Autodesk Inventor part; units mm, degrees
ref_plane "YZ Plane" through (0, 0, 0) normal (1, 0, 0) x (0, 1, 0)
ref_plane "XZ Plane" through (0, 0, 0) normal (0, 1, 0) x (-1, 0, 0)
ref_plane "XY Plane" through (0, 0, 0) normal (0, 0, 1) x (1, 0, 0)
sketch "Sketch1" plane through (0, 0, 0) normal (0, 1, 0) x (-1, 0, 0)
  line L0 (7.5, 75) -> (-7.5, 75)
  line L1 (-7.5, 75) -> (-7.5, -75)
  line L2 (-7.5, -75) -> (7.5, -75)
  line L3 (7.5, -75) -> (7.5, 75)
  line L4 (-7.5, 75) -> (7.5, -75) construction
  line L5 (-7.5, -75) -> (7.5, 75) construction
  line L6 (7.5, -66.5) -> (9.3, -66.5)
  line L7 (13.3, -70.5) -> (13.3, -71)
  line L8 (9.3, -75) -> (7.5, -75)
  line L9 (7.5, -75) -> (7.5, -66.5)
  arc A0 (13.3, -70.5) -> (9.3, -66.5) centre (9.3, -70.5) ccw
  arc A1 (9.3, -75) -> (13.3, -71) centre (9.3, -71) ccw
  line L10 (0, 75) -> (0, -75) construction
  line L11 (-7.5, -66.5) -> (-9.3, -66.5)
  line L12 (-13.3, -70.5) -> (-13.3, -71)
  line L13 (-9.3, -75) -> (-7.5, -75)
  arc A2 (-9.3, -66.5) -> (-13.3, -70.5) centre (-9.3, -70.5) ccw
  arc A3 (-13.3, -71) -> (-9.3, -75) centre (-9.3, -71) ccw
  line L14 (-7.5, 0) -> (7.5, 0) construction
  line L15 (7.5, 66.5) -> (9.3, 66.5)
  line L16 (13.3, 70.5) -> (13.3, 71)
  line L17 (9.3, 75) -> (7.5, 75)
  arc A4 (9.3, 66.5) -> (13.3, 70.5) centre (9.3, 70.5) ccw
  arc A5 (13.3, 71) -> (9.3, 75) centre (9.3, 71) ccw
  arc A6 (-13.3, 70.5) -> (-9.3, 66.5) centre (-9.3, 70.5) ccw
  line L18 (-13.3, 70.5) -> (-13.3, 71)
  arc A7 (-9.3, 75) -> (-13.3, 71) centre (-9.3, 71) ccw
  line L19 (-9.3, 75) -> (-7.5, 75)
  line L20 (-7.5, 66.5) -> (-9.3, 66.5)
  line L21 (7.5, -20.0447) -> (7.5, 20.0447)
  line L22 (7.5, 32.5) -> (22.5, 32.5)
  line L23 (27.5, 27.5) -> (27.5, -27.5)
  line L24 (22.5, -32.5) -> (7.5, -32.5)
  line L25 (7.5, -32.5) -> (7.5, 32.5)
  line L26 (-7.5, 1.5) -> (-14.5, 1.5)
  line L27 (-14.5, 1.5) -> (-14.5, -1.5)
  line L28 (-14.5, -1.5) -> (-7.5, -1.5)
  line L29 (-7.5, -1.5) -> (-7.5, 1.5)
  circle A8 centre (-12.5, 0) radius 0.98
  line L30 (22.5, -32.5) -> (27.5, -27.5)
  line L31 (22.5, 32.5) -> (27.5, 27.5)
  point P0 (0, 0)
  point P1 (0, 0)
  point P2 (13.3, -75)
  point P3 (13.3, -66.5)
  point P4 (0, 0)
  point P5 (27.5, -32.5)
  point P6 (27.5, 32.5)
  point P7 (27.5, 0)
  point P8 (0, 0)
  point P9 (-11, -1.5)
  point P10 (-14.5, 0)
  point P11 (-7.5, 0)
  point P12 (7.5, -32.5)
  dimension "d0" = 150
  dimension "d1" = 15
  dimension "d2" = 5.8
  dimension "d3" = 8.5
  dimension "d4" = 4
  dimension "d5" = 20
  dimension "d6" = 65
  dimension "d7" = 1.96
  dimension "d8" = 3
  dimension "d9" = 7
  dimension "d10" = 5
  dimension "d11" = 5
  dimension "d12" = 5
  dimension "d13" = 5
  dimension "d14" = 5
  dimension "d17" = 1.8
  dimension "d18" = 0.5
  dimension "d19" = 4
  dimension "d20" = 4
extrude "Extrusion1" add sketch "Sketch1" along normal blind 1.57 contours L3 L2 L1 L0 | L17 A5 L16 A4 L15 L3 | L1 L20 A6 L18 A7 L19 | L22 L31 L23 L30 L24 L3 | L1 L13 A3 L12 A2 L11 | L6 A0 L7 A1 L8 L3
properties part number "linefollower_chassy_model"
Model file for the job. Use its own axes, mm. A direction names the side the tool comes from. Round coordinates to 2 decimals unless told otherwise and drop trailing zeros. Order: outer loops, then holes, each group sorted by start corner. A loop starts at its lowest first (then second) coordinate and runs counter-clockwise, first axis right, second up. Notation, with made-up numbers: M 11,48.5 L 55,48.5 A19 cw 55,73.5 Z; hole C 71.5,12.25 d2. An arc over 180 degrees is marked long. Use CSV: the item, a comma, the result in double quotes.
Item 1: Saw through at C-C (z = 30). List the corners of the cut face in (x, y), plus the area to 3 significant figures.
Worked answers:
outline,"M -25,0 L 7.5,0 L 7.5,1.57 L -25,1.57 Z"
area,"51.0 mm²"
Item 2: Probe probe 1 along Z at (x, y) = (-9, 0.8); probe 2 along Z at (x, y) = (-10.5, 0.7); probe 3 along X at (y, z) = (0.5, 37). List the from-to ranges inside material, lowest first.
Worked answers:
probe 1,"-75 to -66.5, -32.5 to 32.5, 66.5 to 75"
probe 2,"-74.82 to -66.68, -32.5 to 32.5, 66.68 to 74.82"
probe 3,"-7.5 to 7.5"
Item 3: Which spindle directions (+Z, -Z, +X, -X, +Y, -Y) get a long thin tool onto all of the face, cutting with end or side? Do faces 4 (the face through (12.159, 0.774, -67.703)), 5 (the face through (-12.159, 0.774, -73.797)), 6 (the face through (-12.097, 0.774, -67.641)). Say none if no direction does.
Worked answers:
face 4,"+X, +Y, -Y"
face 5,"-Z, -X, +Y, -Y"
face 6,"-X, +Y, -Y"
Item 4: Saw through at B-B (z = 51.5). List the corners of the cut face in (x, y), plus the area to 4 significant figures.
Worked answers:
outline,"M -7.5,0 L 7.5,0 L 7.5,1.57 L -7.5,1.57 Z"
area,"23.55 mm²"
Item 5: Pin check, flat tips, straight feed: pin 1 (0.6 mm diameter, centred on y = 1, z = -71, fed in from -X); pin 2 (0.8 mm diameter, centred on y = 0.5, z = -18.5, fed in from +X); pin 3 (0.5 mm diameter, centred on y = 1, z = 43.5, fed in from -X). Stop position of each tip, or through.
Worked answers:
pin 1,"x = -13.3"
pin 2,"x = 7.5"
pin 3,"x = -7.5"
Item 6: Pull direction Z, two halves, no side cores. Call faces 1 (the face through (12.159, 0.774, 73.797)), 2 (the face through (12.097, 0.774, 67.641)), 3 (the face through (-25, 1, -30)): released by +Z, released by -Z, zero draft, split by the parting line, or undercut.
Worked answers:
face 1,"released by +Z"
face 2,"undercut"
face 3,"released by -Z"
Item 7: Saw through at A-A (y = 0.7). List the corners of the cut face in (x, z), plus the area to 3 significant figures.
Worked answers:
outline,"M -27.5,-27.5 L -22.5,-32.5 L -7.5,-32.5 L -7.5,-66.5 L -9.3,-66.5 A4 ccw -13.3,-70.5 L -13.3,-71 A4 ccw -9.3,-75 L 9.3,-75 A4 ccw 13.3,-71 L 13.3,-70.5 A4 ccw 9.3,-66.5 L 7.5,-66.5 L 7.5,66.5 L 9.3,66.5 A4 ccw 13.3,70.5 L 13.3,71 A4 ccw 9.3,75 L -9.3,75 A4 ccw -13.3,71 L -13.3,70.5 A4 ccw -9.3,66.5 L -7.5,66.5 L -7.5,32.5 L -22.5,32.5 L -27.5,27.5 Z"
area,"3,690 mm²"
